Part model, mm, in its own coordinate system. Face numbers are marked on the shaded views. A direction names the side the tool comes from. Round coordinates to 2 decimals unless told otherwise and drop trailing zeros. Order: outer loops, then holes, each group sorted by start corner. A loop starts at its lowest first (then second) coordinate and runs counter-clockwise, first axis right, second up. Notation, with made-up numbers: (13.25, 28) - (17.25, 28) arc R21 cw to (17.25, 41) - close; hole circle Ø6 at (27, 41.25). An arc over 180 degrees is marked (long way). Answer as a JSON object with one key per item and string values.
```python
from build123d import *

# Parameters (mm, degrees)
CROQUIS1_R              = 3
SALIENTE_EXTRUIR1_DEPTH = 80
CROQUIS2_W              = 5.531234996
CROQUIS2_H              = 1
CORTAR_EXTRUIR1_REACH   = 83.112
CORTAR_EXTRUIR1_START   = 1
CROQUIS3_W              = 6
CROQUIS3_H              = 6
CORTAR_EXTRUIR3_REACH   = 84.112
CORTAR_EXTRUIR3_START   = -2
CROQUIS3_2_W            = 6
CROQUIS3_2_H            = 8
CORTAR_EXTRUIR4_REACH   = 84.112
CORTAR_EXTRUIR4_START   = 2
CROQUIS3_4_W            = 6
CROQUIS3_4_H            = 8
CHAFL_N1_SIZE           = 0.5


with BuildPart() as part:
    # Croquis1 → Saliente-Extruir1 (new body)
    with BuildSketch(Plane(origin=(0, 0, 0), x_dir=(1, 0, 0), z_dir=(0, 1, 0))):
        with Locations(Location((0, 0, 0), (0, 0, 270))):
            Circle(CROQUIS1_R)
    extrude(amount=SALIENTE_EXTRUIR1_DEPTH)

    # Croquis2 → Cortar-Revoluci_n1 (revolve, cut)
    with BuildSketch(Plane.XY, mode=Mode.PRIVATE) as cortar_revoluci_n1_sk:
        with Locations((5.565617498, 77.5)):
            Rectangle(CROQUIS2_W, CROQUIS2_H)
        with Locations((5.565617498, 2.5)):
            Rectangle(CROQUIS2_W, CROQUIS2_H)
    revolve(cortar_revoluci_n1_sk.sketch.rotate(Axis((0, 80, 0), (0, -1, 0)), 90), axis=Axis((0, 80, 0), (0, -1, 0)), mode=Mode.SUBTRACT)

    # Croquis3 → Cortar-Extruir1 (cut, up to next)
    with BuildSketch(Plane(origin=(0, 0, 0), x_dir=(0, 0, -1), z_dir=(1, 0, 0)).offset(CORTAR_EXTRUIR1_START), mode=Mode.PRIVATE) as cortar_extruir1_sk1:
        with Locations((0, 62)):
            Rectangle(CROQUIS3_W, CROQUIS3_H)
    cortar_extruir1_tool1 = extrude(cortar_extruir1_sk1.sketch, amount=CORTAR_EXTRUIR1_REACH, mode=Mode.PRIVATE) & part.part
    add(cortar_extruir1_tool1.solids().sort_by_distance((1, 62, 0))[0], mode=Mode.SUBTRACT)

    # Croquis3_2 → Cortar-Extruir3 (cut, up to next)
    with BuildSketch(Plane(origin=(0, 0, 0), x_dir=(0, 0, -1), z_dir=(1, 0, 0)).offset(CORTAR_EXTRUIR3_START), mode=Mode.PRIVATE) as cortar_extruir3_sk1:
        with Locations((0, 39)):
            Rectangle(CROQUIS3_2_W, CROQUIS3_2_H)
    cortar_extruir3_tool1 = extrude(cortar_extruir3_sk1.sketch, amount=-CORTAR_EXTRUIR3_REACH, mode=Mode.PRIVATE) & part.part
    add(cortar_extruir3_tool1.solids().sort_by_distance((-2, 39, 0))[0], mode=Mode.SUBTRACT)

    # Croquis3_4 → Cortar-Extruir4 (cut, up to next)
    with BuildSketch(Plane(origin=(0, 0, 0), x_dir=(0, 0, -1), z_dir=(1, 0, 0)).offset(CORTAR_EXTRUIR4_START), mode=Mode.PRIVATE) as cortar_extruir4_sk1:
        with Locations((0, 39)):
            Rectangle(CROQUIS3_4_W, CROQUIS3_4_H)
    cortar_extruir4_tool1 = extrude(cortar_extruir4_sk1.sketch, amount=CORTAR_EXTRUIR4_REACH, mode=Mode.PRIVATE) & part.part
    add(cortar_extruir4_tool1.solids().sort_by_distance((2, 39, 0))[0], mode=Mode.SUBTRACT)

    # Chafl_n1
    chafl_n1_edges = [part.edges().sort_by_distance(p)[0] for p in [
        (0, 0, -3),
        (0, 80, -3),
    ]]
    chamfer(chafl_n1_edges, length=CHAFL_N1_SIZE)


solid = part.part
```
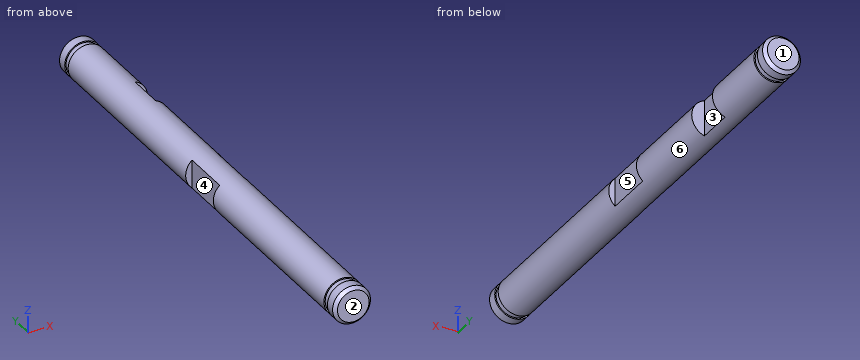
Item 1: Cut at B-B (y = 37.5). Write the cut outline in (x, z), plus the area to 3 significant figures.
Taken from the geometry:
{"outline": "(-2, -2.24) arc R3 ccw to (2, -2.24) - (2, 2.24) arc R3 ccw to (-2, 2.24) - close", "area": "22.1 mm2"}
Item 2: Drop flat-ended pins along their axis: P1, Ø2, axis at y = 40, z = -0.5, coming from the -X side; P2, Ø0.5, axis at x = 2.5, z = -0.5, coming from the -Y side; P3, Ø1, axis at x = -1, y = 58, coming from the -Z side; P4, Ø2, axis at y = 37, z = 0, coming from the +X side. Give the stop position or say it passes through.
Taken from the geometry:
{"P1": "x = -2", "P2": "y = 0", "P3": "z = -2.96", "P4": "x = 2"}
Item 3: Cut at A-A (y = 63). Write the cut outline in (x, z), plus the area to 3 significant figures.
Taken from the geometry:
{"outline": "(1, -2.83) - (1, 2.83) arc R3 ccw (long way) to start", "area": "20.0 mm2"}
Item 4: Two-plate mould, pull along Y, no slides. Class the marked faces 1, 2 and 3: pulls with the +Y half, pulls with the -Y half, needs draft (parallel to the pull), parting line crosses it, or undercut.
Taken from the geometry:
{"face 1": "pulls with the +Y half", "face 2": "pulls with the -Y half", "face 3": "undercut"}
Item 5: Probe L1, parallel to Y at x = 1.35, z = 1.7; L2, parallel to Y at x = 2.5, z = -0.35; L3, parallel to Y at x = -2.4, z = 0.6. List the from-to ranges inside material, lowest first. Write a range as from..to.
Taken from the geometry:
{"L1": "0..59, 65..80", "L2": "0.02..35, 43..59, 65..79.98", "L3": "0..35, 43..80"}
Item 6: Cut at C-C (y = 53). Write the cut outline in (x, z), plus the area to 3 significant figures.
Taken from the geometry:
{"outline": "circle Ø6 at (0, 0)", "area": "28.3 mm2"}
Item 7: Tool access for the marked faces 4, 5 and 6: list every direction of +Z, -Z, +X, -X, +Y, -Y with a clear straight run to the whole face (end or side of a thin tool).
Taken from the geometry:
{"face 4": "+Z, -Z, -X", "face 5": "+Z, -Z, +X", "face 6": "+Y, -Y"}
